Read the model definition and answer for the solid it produces. Units are mm, in the model's axes. Give positions to 0.01 mm unless a question says otherwise; leave off trailing zeros. Order: outer loops, then holes, each group sorted by start corner. A loop starts at its lowest first (then second) coordinate and runs counter-clockwise, first axis right, second up. Notation, with made-up numbers: (61, 51) - (105, 51) arc R8 cw to (105, 57) - close; hole circle Ø9 at (55.5, -32.75). An arc over 180 degrees is marked (long way). Write each question's results on one line, items separated by ' | '. Start each with the question number.
Q1. Find the intervals of material crossed by line 1 along Z through (x, y) = (94.5, 0.6); line 2 along X through (y, z) = (1.15, -2.5); line 3 along Z through (x, y) = (45.5, 1.65), in increasing order. Write a range as from..to.
Q2. Flat-ended cylindrical pins translate along their axes: P1, Ø1.6, axis at y = 1.5, z = -87.5, coming from the +X side; P2, Ø2, axis at x = 107.02, z = -83.5, coming from the -Y side; P3, Ø1.5, axis at y = 2, z = 40.5, coming from the +X side; P4, Ø0.9, axis at x = 215, y = 1.5, coming from the +Z side. Find the tip coordinate at first contact, or state that the pin passes through.
Q3. Find section B-B on y = 2.45. Count the separate pieces of the cut face and the enclosed holes in it, and give its area (3 significant figures).
Q4. Find section A-A on x = 96. Give the vertices of the cut face in (y, z), and give its area (3 significant figures).
from build123d import *

# Parameters (mm, degrees)
ESTRUSIONE_ESTRUSIONE1_DEPTH  = 3
FORO_FILETTATO_M3X0_5_1_D     = 2.5
FORO_FILETTATO_M3X0_5_1_DEPTH = 7.5
FORO_FILETTATO_M3X0_5_1_TIP   = 0.751075774
SCHIZZO4_W                    = 89.03043591
SCHIZZO4_H                    = 2
TAGLIO_ESTRUSIONE2_DEPTH      = 10
FORO_FILETTATO_M3X0_5_7_D     = 2.5
SCHIZZO29_W                   = 5
SCHIZZO29_H                   = 2
TAGLIO_ESTRUSIONE13_DEPTH     = 10
SCHIZZO7_W                    = 2
SCHIZZO7_H                    = 47.5
TAGLIO_ESTRUSIONE5_DEPTH      = 10
SCHIZZO10_W                   = 2
SCHIZZO10_H                   = 38.172865154
TAGLIO_ESTRUSIONE6_DEPTH      = 262.897403576
FORO_FILETTATO_M3X0_5_2_D     = 2.5
SCHIZZO17_W                   = 25
SCHIZZO17_H                   = 2
SCHIZZO17_W_2                 = 2
SCHIZZO17_H_2                 = 20
SCHIZZO17_H_3                 = 25
TAGLIO_ESTRUSIONE9_DEPTH      = 10
SCHIZZO18_W                   = 70
SCHIZZO18_H                   = 2
TAGLIO_ESTRUSIONE10_DEPTH     = 10
FORO_FILETTATO_M3X0_5_3_D     = 2.5
SCHIZZO25_W                   = 2
SCHIZZO25_H                   = 30
TAGLIO_ESTRUSIONE11_DEPTH     = 10
FORO_FILETTATO_M3X0_5_6_D     = 2.5
SCHIZZO36_W                   = 30
SCHIZZO36_H                   = 15
TAGLIO_ESTRUSIONE15_DEPTH     = 10
SCHIZZO37_W                   = 35
SCHIZZO37_H                   = 15
TAGLIO_ESTRUSIONE16_DEPTH     = 10
SCHIZZO38_W                   = 45
SCHIZZO38_H                   = 30
TAGLIO_ESTRUSIONE17_DEPTH     = 10
FORO_FILETTATO_M3X0_5_9_D     = 2.5
RACCORDO1_R                   = 8
RACCORDO2_R                   = 10
RACCORDO3_R                   = 5
FORO_PER_VITE_M3_1_D          = 3.4


with BuildPart() as part:
    # Schizzo1 → Estrusione-Estrusione1 (new body)
    with BuildSketch(Plane(origin=(0, 0, 0), x_dir=(1, 0, 0), z_dir=(0, 1, 0))):
        Polygon((70, 67.5), (70, 92.5), (185.052105959, 92.5), (228.353376148, 74.033119315), (245, 30), (245, -30), (228.353376148, -74.033119315), (185.052105959, -92.5), (70, -92.5), (70, -67.5), (0, -67.5), (0, 67.5), align=None)
    extrude(amount=ESTRUSIONE_ESTRUSIONE1_DEPTH)

    # Foro filettato M3x0.5-1
    with Locations(Plane(origin=(0, 3, 0), x_dir=(1, 0, 0), z_dir=(0, 1, 0))):
        with Locations((224.430485984, 70.270415253), (240, 29.086432577), (240, -29.086432577), (224.430485984, -70.270415253), (184.03043591, -87.5), (184.03043591, 87.5), (75, 87.5), (75, -87.5), (5, -62.5), (5, 62.5)):
            Hole(FORO_FILETTATO_M3X0_5_1_D / 2, depth=FORO_FILETTATO_M3X0_5_1_DEPTH)
            with Locations((0, 0, -(FORO_FILETTATO_M3X0_5_1_DEPTH + FORO_FILETTATO_M3X0_5_1_TIP / 2))):  # 118° drill point
                Cone(0, FORO_FILETTATO_M3X0_5_1_D / 2, FORO_FILETTATO_M3X0_5_1_TIP, mode=Mode.SUBTRACT)

    # Schizzo4 → Taglio-Estrusione2 (cut)
    with BuildSketch(Plane(origin=(0, 3, 0), x_dir=(1, 0, 0), z_dir=(0, 1, 0))):
        with Locations((129.515217955, -87.5)):
            Rectangle(SCHIZZO4_W, SCHIZZO4_H)
        Polygon((235.52839554, 38.086696659), (227.03131331, 60.562907992), (228.902090444, 61.27015117), (237.399172674, 38.793939838), align=None)
        with Locations((129.515217955, 87.5)):
            Rectangle(SCHIZZO4_W, SCHIZZO4_H)
        Polygon((215.624354877, 75.113147429), (193.62114505, 84.496951848), (192.836567017, 82.657267824), (214.839776844, 73.273463404), align=None)
        Polygon((192.836567017, -82.657267824), (214.839776844, -73.273463404), (215.624354877, -75.113147429), (193.62114505, -84.496951848), align=None)
        Polygon((227.03131331, -60.562907992), (235.52839554, -38.086696659), (237.399172674, -38.793939838), (228.902090444, -61.27015117), align=None)
    extrude(amount=-TAGLIO_ESTRUSIONE2_DEPTH, mode=Mode.SUBTRACT)

    # Foro filettato M3x0.5-7 (through all)
    with Locations(Plane(origin=(0, 3, 0), x_dir=(1, 0, 0), z_dir=(0, 1, 0))):
        with Locations((107.015217955, -83.5), (152.015217955, -83.5)):
            foro_filettato_m3x0_5_7 = Hole(FORO_FILETTATO_M3X0_5_7_D / 2)

    # Schizzo29 → Taglio-Estrusione13 (cut)
    with BuildSketch(Plane(origin=(0, 3, 0), x_dir=(1, 0, 0), z_dir=(0, 1, 0))):
        with Locations((82.5, -87.5)):
            Rectangle(SCHIZZO29_W, SCHIZZO29_H)
        with Locations((176.53043591, -87.5)):
            Rectangle(SCHIZZO29_W, SCHIZZO29_H)
    taglio_estrusione13 = extrude(amount=-TAGLIO_ESTRUSIONE13_DEPTH, mode=Mode.SUBTRACT)

    # Specchia2: Foro filettato M3x0.5-7, Taglio-Estrusione13 across plane
    add(foro_filettato_m3x0_5_7.mirror(Plane.XY), mode=Mode.SUBTRACT)
    add(taglio_estrusione13.mirror(Plane.XY), mode=Mode.SUBTRACT)

    # Schizzo7 → Taglio-Estrusione5 (cut)
    with BuildSketch(Plane(origin=(0, 3, 0), x_dir=(1, 0, 0), z_dir=(0, 1, 0))):
        with Locations((5, 28.75)):
            Rectangle(SCHIZZO7_W, SCHIZZO7_H)
        with Locations((5, -28.75)):
            Rectangle(SCHIZZO7_W, SCHIZZO7_H)
    extrude(amount=-TAGLIO_ESTRUSIONE5_DEPTH, mode=Mode.SUBTRACT)

    # Schizzo10 → Taglio-Estrusione6 (cut, through all)
    with BuildSketch(Plane(origin=(0, 3, 0), x_dir=(1, 0, 0), z_dir=(0, 1, 0))):
        with Locations((240, 0)):
            Rectangle(SCHIZZO10_W, SCHIZZO10_H)
    extrude(amount=-TAGLIO_ESTRUSIONE6_DEPTH, mode=Mode.SUBTRACT)

    # Foro filettato M3x0.5-2 (through all)
    with Locations(Plane(origin=(0, 3, 0), x_dir=(1, 0, 0), z_dir=(0, 1, 0))):
        with Locations((13, 54.5), (13, -54.5), (58, -54.5), (58, 54.5)):
            Hole(FORO_FILETTATO_M3X0_5_2_D / 2)

    # Schizzo17 → Taglio-Estrusione9 (cut)
    with BuildSketch(Plane(origin=(0, 3, 0), x_dir=(1, 0, 0), z_dir=(0, 1, 0))):
        with Locations((35.5, -54.5)):
            Rectangle(SCHIZZO17_W, SCHIZZO17_H)
        with Locations((13, -34.5)):
            Rectangle(SCHIZZO17_W_2, SCHIZZO17_H_2)
        with Locations((13, 34.5)):
            Rectangle(SCHIZZO17_W_2, SCHIZZO17_H_2)
        with Locations((35.5, 54.5)):
            Rectangle(SCHIZZO17_W, SCHIZZO17_H)
        with Locations((13, 0)):
            Rectangle(SCHIZZO17_W_2, SCHIZZO17_H_3)
    extrude(amount=-TAGLIO_ESTRUSIONE9_DEPTH, mode=Mode.SUBTRACT)

    # Schizzo18 → Taglio-Estrusione10 (cut)
    with BuildSketch(Plane(origin=(0, 3, 0), x_dir=(1, 0, 0), z_dir=(0, 1, 0))):
        with Locations((113, 78.5)):
            Rectangle(SCHIZZO18_W, SCHIZZO18_H)
        with Locations((113, -78.5)):
            Rectangle(SCHIZZO18_W, SCHIZZO18_H)
    extrude(amount=-TAGLIO_ESTRUSIONE10_DEPTH, mode=Mode.SUBTRACT)

    # Foro filettato M3x0.5-3 (through all)
    with Locations(Plane(origin=(0, 3, 0), x_dir=(1, 0, 0), z_dir=(0, 1, 0))):
        with Locations((230, 26.586432577), (230, -26.586432577)):
            Hole(FORO_FILETTATO_M3X0_5_3_D / 2)

    # Schizzo25 → Taglio-Estrusione11 (cut)
    with BuildSketch(Plane(origin=(0, 3, 0), x_dir=(1, 0, 0), z_dir=(0, 1, 0))):
        with Locations((230, 0)):
            Rectangle(SCHIZZO25_W, SCHIZZO25_H)
    extrude(amount=-TAGLIO_ESTRUSIONE11_DEPTH, mode=Mode.SUBTRACT)

    # Foro filettato M3x0.5-6 (through all)
    with Locations(Plane(origin=(0, 3, 0), x_dir=(1, 0, 0), z_dir=(0, 1, 0))):
        with Locations((73, 58.5), (190, 58.5), (190, -58.5), (73, -58.5)):
            Hole(FORO_FILETTATO_M3X0_5_6_D / 2)

    # Schizzo36 → Taglio-Estrusione15 (cut)
    with BuildSketch(Plane(origin=(0, 3, 0), x_dir=(1, 0, 0), z_dir=(0, 1, 0))):
        with Locations((210, 0)):
            Rectangle(SCHIZZO36_W, SCHIZZO36_H)
    extrude(amount=-TAGLIO_ESTRUSIONE15_DEPTH, mode=Mode.SUBTRACT)

    # Schizzo37 → Taglio-Estrusione16 (cut)
    with BuildSketch(Plane(origin=(0, 3, 0), x_dir=(1, 0, 0), z_dir=(0, 1, 0))):
        with Locations((37.5, 0)):
            Rectangle(SCHIZZO37_W, SCHIZZO37_H)
    extrude(amount=-TAGLIO_ESTRUSIONE16_DEPTH, mode=Mode.SUBTRACT)

    # Schizzo38 → Taglio-Estrusione17 (cut)
    with BuildSketch(Plane(origin=(0, 3, 0), x_dir=(1, 0, 0), z_dir=(0, 1, 0))):
        with Locations((122.5, 35)):
            Rectangle(SCHIZZO38_W, SCHIZZO38_H)
        with Locations((122.5, -35)):
            Rectangle(SCHIZZO38_W, SCHIZZO38_H)
    extrude(amount=-TAGLIO_ESTRUSIONE17_DEPTH, mode=Mode.SUBTRACT)

    # Foro filettato M3x0.5-9 (through all)
    with Locations(Plane(origin=(0, 3, 0), x_dir=(1, 0, 0), z_dir=(0, 1, 0))):
        with Locations((20.49, -47.01), (53.51, -47.01), (53.51, -13.99), (20.49, -13.99)):
            Hole(FORO_FILETTATO_M3X0_5_9_D / 2)

    # Raccordo1
    raccordo1_edges = [part.edges().sort_by_distance(p)[0] for p in [
        (0, 1.5, -67.5),
        (70, 1.5, -67.5),
        (70, 1.5, -92.5),
        (70, 1.5, 92.5),
        (70, 1.5, 67.5),
        (0, 1.5, 67.5),
    ]]
    fillet(raccordo1_edges, radius=RACCORDO1_R)

    # Raccordo2
    raccordo2_edges = [part.edges().sort_by_distance(p)[0] for p in [
        (185.052105959, 1.5, -92.5),
        (228.353376148, 1.5, -74.033119315),
        (245, 1.5, -30),
        (245, 1.5, 30),
        (228.353376148, 1.5, 74.033119315),
        (185.052105959, 1.5, 92.5),
    ]]
    fillet(raccordo2_edges, radius=RACCORDO2_R)

    # Raccordo3
    raccordo3_edges = [part.edges().sort_by_distance(p)[0] for p in [
        (195, 1.5, 7.5),
        (195, 1.5, -7.5),
        (225, 1.5, -7.5),
        (225, 1.5, 7.5),
        (20, 1.5, 7.5),
        (20, 1.5, -7.5),
        (55, 1.5, -7.5),
        (55, 1.5, 7.5),
        (100, 1.5, -20),
        (100, 1.5, -50),
        (145, 1.5, -50),
        (145, 1.5, -20),
        (100, 1.5, 50),
        (100, 1.5, 20),
        (145, 1.5, 20),
        (145, 1.5, 50),
    ]]
    fillet(raccordo3_edges, radius=RACCORDO3_R)

    # Foro per Vite M3-1 (through all)
    with Locations(Plane(origin=(0, 3, 0), x_dir=(1, 0, 0), z_dir=(0, 1, 0))):
        with Locations((83, 70), (103, 70), (103, -70), (83, -70)):
            Hole(FORO_PER_VITE_M3_1_D / 2)


solid = part.part
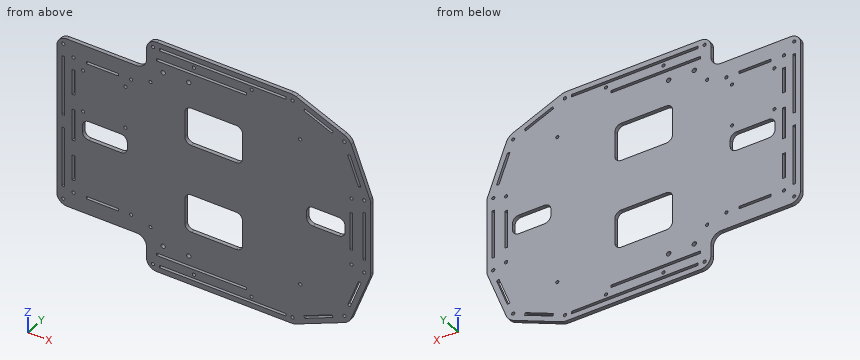
Working result:
1) line 1: -92.5..-88.5, -86.5..-79.5, -77.5..77.5, 79.5..86.5, 88.5..92.5 | line 2: 0..12, 14..20, 55..195, 225..229, 231..239, 241..245 | line 3: -67.5..-55.5, -53.5..-7.5, 7.5..53.5, 55.5..67.5
2) P1: x = 198.65 | P2: through | P3: x = 241.31 | P4: z = 79.92
3) separate pieces: 1 | enclosed holes: 53 | area: 34,500 mm²
4) outline: (0, -92.5) - (3, -92.5) - (3, -88.5) - (0, -88.5) - close; (0, -86.5) - (3, -86.5) - (3, -79.5) - (0, -79.5) - close; (0, -77.5) - (3, -77.5) - (3, 77.5) - (0, 77.5) - close; (0, 79.5) - (3, 79.5) - (3, 86.5) - (0, 86.5) - close; (0, 88.5) - (3, 88.5) - (3, 92.5) - (0, 92.5) - close | area: 531 mm²
